For this review, take the finished solid that the model builds, in its own axes (mm). Face numbers are marked on the shaded views. Give positions to 0.01 mm unless a question says otherwise; leave off trailing zeros. Write each loop counter-clockwise with the first axis right and the second up, starting at its lowest first coordinate (ties: lowest second). Pieces come first, ordered by that corner, then holes. Notation, with made-up numbers: (-7.75, 89) -> (26.25, 89) arc R19 ccw to (26.25, 94) -> close; hole circle Ø2 at (15.25, 86.5). An arc over 180 degrees is marked (long way). Return JSON: item names as keys, results as strings.
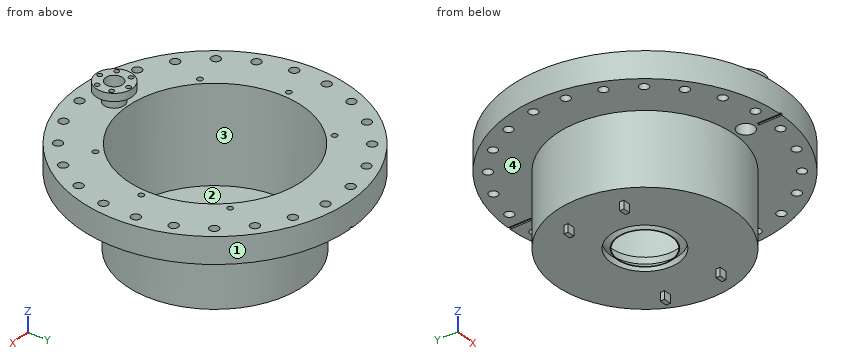
from build123d import *

# Parameters (mm, degrees)
SKETCH1_R                   = 83.5
SKETCH1_R_2                 = 82.5
EXTRUDE1_DEPTH              = 67.31
SKETCH2_R                   = 127
SKETCH2_R_2                 = 82.5
EXTRUDE2_DEPTH              = 24.511
SKETCH3_R                   = 4.2
CUT_EXTRUDE1_DEPTH          = 24.511
CIRPATTERN1_COUNT           = 24
SKETCH4_R                   = 83.5
SKETCH4_R_2                 = 32.2
EXTRUDE3_DEPTH              = 2
SKETCH13_R                  = 7.9375
EXTRUDE4_DEPTH              = 110.601
SKETCH14_R                  = 9.4996
SKETCH14_R_2                = 7.9375
EXTRUDE5_DEPTH              = 17.78
SKETCH15_R                  = 16.891
SKETCH15_R_2                = 7.9375
EXTRUDE6_DEPTH              = 7.239
SKETCH16_R                  = 2.1844
EXTRUDE7_DEPTH              = 7.239
CIRPATTERN2_COUNT           = 6
SKETCH17_W                  = 6.858832098
SKETCH17_H                  = 3.977015868
EXTRUDE8_DEPTH              = 7.62
MIRROR4_COPY_1_SKETCH_W     = 6.858832098
MIRROR4_COPY_1_SKETCH_H     = 3.977015868
MIRROR4_COPY_1_DEPTH        = 7.62
F_1_4_20_TAPPED_HOLE1_D     = 5.1054
F_1_4_20_TAPPED_HOLE1_DEPTH = 12.7
F_1_4_20_TAPPED_HOLE1_TIP   = 1.533816902
SKETCH21_W                  = 2.54
SKETCH21_H                  = 27.464757855
EXTRUDE9_DEPTH              = 1.27


with BuildPart() as part:
    # Sketch1 → Extrude1 (new body)
    with BuildSketch(Plane.XY):
        Circle(SKETCH1_R)
        Circle(SKETCH1_R_2, mode=Mode.SUBTRACT)
    extrude(amount=-EXTRUDE1_DEPTH)

    # Sketch2 → Extrude2 (add)
    with BuildSketch(Plane.XY):
        Circle(SKETCH2_R)
        Circle(SKETCH2_R_2, mode=Mode.SUBTRACT)
    extrude(amount=EXTRUDE2_DEPTH)

    # Sketch3 → Cut-Extrude1 (cut)
    with BuildSketch(Plane.XY.offset(24.511)):
        with Locations((15.131327149, -114.933840422)):
            Circle(SKETCH3_R)
    cut_extrude1 = extrude(amount=-CUT_EXTRUDE1_DEPTH, mode=Mode.SUBTRACT)

    # CirPattern1: Cut-Extrude1 ×24 about axis
    cirpattern1_axis = Axis((0, 0, 0), (0, 0, 1))
    for i in range(1, CIRPATTERN1_COUNT):
        add(cut_extrude1.rotate(cirpattern1_axis, i * 360 / CIRPATTERN1_COUNT), mode=Mode.SUBTRACT)

    # Sketch4 → Extrude3 (add)
    with BuildSketch(Plane(origin=(0, 0, -67.31), x_dir=(-1, 0, 0), z_dir=(0, 0, -1))):
        Circle(SKETCH4_R)
        Circle(SKETCH4_R_2, mode=Mode.SUBTRACT)
    extrude(amount=-EXTRUDE3_DEPTH)

    # Sketch5 → Revolve1 (revolve)
    with BuildSketch(Plane(origin=(0, 0, 0), x_dir=(1, 0, 0), z_dir=(0, 1, 0))):
        Polygon((-32.2, 67.31), (-32.2, 55.31), (-31, 55.31), (-31, 61.31), (-25, 67.31), align=None)
    revolve(axis=Axis((0, 0, 0), (0, 0, -1)))

    # Sketch11 → Cut-Revolve1 (revolve, cut)
    with BuildSketch(Plane(origin=(0, 0, 0), x_dir=(1, 0, 0), z_dir=(0, 1, 0))):
        Polygon((-31.7, 67.31), (-31.7, 61.317106781), (-25.707106781, 67.31), align=None)
    revolve(axis=Axis((0, 0, 0), (0, 0, -1)), mode=Mode.SUBTRACT)

    # Sketch13 → Extrude4 (cut, through all)
    with BuildSketch(Plane.XY.offset(42.291)):
        with Locations((0, -94.25)):
            Circle(SKETCH13_R)
    extrude(amount=-EXTRUDE4_DEPTH, mode=Mode.SUBTRACT)

    # Sketch14 → Extrude5 (add)
    with BuildSketch(Plane.XY.offset(42.291)):
        with Locations((0, -94.25)):
            Circle(SKETCH14_R)
        with Locations((0, -94.25)):
            Circle(SKETCH14_R_2, mode=Mode.SUBTRACT)
    extrude(amount=-EXTRUDE5_DEPTH)

    # Sketch15 → Extrude6 (add)
    with BuildSketch(Plane.XY.offset(42.291)):
        with Locations((0, -94.25)):
            Circle(SKETCH15_R)
        with Locations((0, -94.25)):
            Circle(SKETCH15_R_2, mode=Mode.SUBTRACT)
    extrude(amount=-EXTRUDE6_DEPTH)

    # Sketch16 → Extrude7 (cut)
    with BuildSketch(Plane.XY.offset(42.291)):
        with Locations((0, -80.7626)):
            Circle(SKETCH16_R)
    extrude7 = extrude(amount=-EXTRUDE7_DEPTH, mode=Mode.SUBTRACT)

    # CirPattern2: Extrude7 ×6 about axis
    cirpattern2_axis = Axis((0, -94.25, 0), (0, 0, 1))
    for i in range(1, CIRPATTERN2_COUNT):
        add(extrude7.rotate(cirpattern2_axis, i * 360 / CIRPATTERN2_COUNT), mode=Mode.SUBTRACT)

    # Sketch17 → Extrude8 (add)
    with BuildSketch(Plane(origin=(0, 0, -67.31), x_dir=(-1, 0, 0), z_dir=(0, 0, -1))):
        with Locations((-58, -26)):
            Rectangle(SKETCH17_W, SKETCH17_H)
    extrude8 = extrude(amount=EXTRUDE8_DEPTH)

    # Mirror3: Extrude8 across plane
    add(extrude8.mirror(Plane.ZX))

    # Mirror4: Extrude8 across plane
    add(extrude8.mirror(Plane(origin=(0, 0, 0), x_dir=(0, 0, 1), z_dir=(1, 0, 0))))

    # Mirror4 copy 1 sketch → Mirror4 copy 1 (add)
    with BuildSketch(Plane(origin=(0, 0, -67.31), x_dir=(1, 0, 0), z_dir=(0, 0, -1))):
        with Locations((-58, -26)):
            Rectangle(MIRROR4_COPY_1_SKETCH_W, MIRROR4_COPY_1_SKETCH_H)
    extrude(amount=MIRROR4_COPY_1_DEPTH)

    # 1/4-20 Tapped Hole1
    with Locations(Plane(origin=(62.861792847, -62.861792847, 24.511), x_dir=(1, 0, 0), z_dir=(0, 0, 1))):
        with Locations((0, 0), (-125.723585694, 0), (-151.761792847, 62.861792847), (-125.723585694, 125.723585694), (0, 125.723585694), (26.038207153, 62.861792847)):
            Hole(F_1_4_20_TAPPED_HOLE1_D / 2, depth=F_1_4_20_TAPPED_HOLE1_DEPTH)
            with Locations((0, 0, -(F_1_4_20_TAPPED_HOLE1_DEPTH + F_1_4_20_TAPPED_HOLE1_TIP / 2))):  # 118° drill point
                Cone(0, F_1_4_20_TAPPED_HOLE1_D / 2, F_1_4_20_TAPPED_HOLE1_TIP, mode=Mode.SUBTRACT)

    # Sketch21 → Extrude9 (cut)
    with BuildSketch(Plane(origin=(0, 0, 0), x_dir=(-1, 0, 0), z_dir=(0, 0, -1))):
        with Locations((0, -119.254869633)):
            Rectangle(SKETCH21_W, SKETCH21_H)
        with Locations((0, 119.254869633)):
            Rectangle(SKETCH21_W, SKETCH21_H)
    extrude(amount=-EXTRUDE9_DEPTH, mode=Mode.SUBTRACT)


solid = part.part
1. The part is to be moulded in two halves that separate along Y. For the marked faces 1, 2, 3 and 4, say which applies: +Y half, -Y half, draft (parallel to the pull), parting line (faces both ways), or undercut.
Results found:
{"face 1": "parting line", "face 2": "undercut", "face 3": "undercut", "face 4": "draft"}
2. Add section A-A, the plane z = -18. State the section outline as (x, y) points.
Results found:
{"outline": "circle Ø167 at (0, 0); hole circle Ø165 at (0, 0)"}
3. To check wall thickness, follow probe 1 along Z at (x, y) = (62, 85.5); probe 2 along Z at (x, y) = (14, 51); probe 3 along X at (y, z) = (-3, -45). State the ranges of each line that lie inside material, in increasing order.
Results found:
{"probe 1": "z = 0 to 24.51", "probe 2": "z = -67.31 to -65.31", "probe 3": "x = -83.45 to -82.45, 82.45 to 83.45"}
4. For pin 1 (10 mm diameter, centred on x = -1, y = -90, fed in from -Z); pin 2 (3 mm diameter, centred on y = 25.5, z = -69.5, fed in from -X); pin 3 (9.5 mm diameter, centred on x = -70.57, y = 91.97, fed in from +Z), all flat-tipped, find the tip position at first contact; note any pin that passes through.
Results found:
{"pin 1": "stops at z = 0", "pin 2": "stops at x = -61.43", "pin 3": "stops at z = 24.51"}
